Input: part model. Units: mm. Frame: model coordinates. Face numbers are marked on the shaded views. A direction names the side the tool comes from. Give positions to 0.01 mm unless a question says otherwise; leave off trailing zeros. Use a Markdown table: item, result. Add a question column.
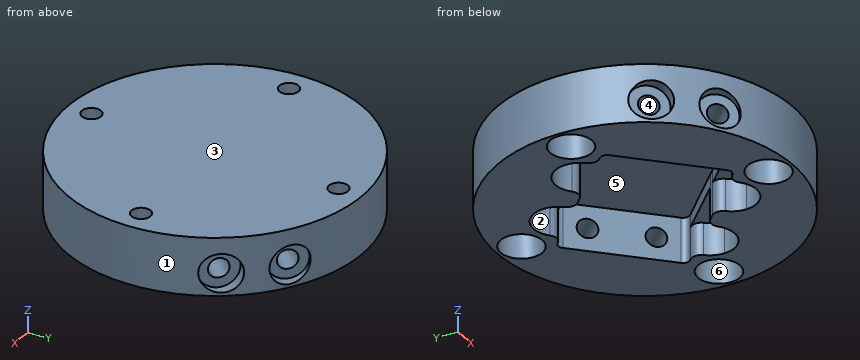
from build123d import *

# Parameters (mm, degrees)
SKETCH_1_R               = 23
SKETCH_1_R_2             = 1.5
EXTRUDE_1_DEPTH          = 7
FILLET_1_R               = 1.5
FILLET_2_R               = 1.5
EXTRUDE_2_DEPTH          = 2
FILLET_3_R               = 1
SKETCH_4_R               = 3.25
SKETCH_4_R_2             = 1.5
CUT_EXTRUDE_1_DEPTH      = 4
SKETCH_5_R               = 23
SKETCH_5_R_2             = 1.5
EXTRUDE_3_DEPTH          = 2
CUT_EXTRUDE_2_DEPTH      = 47.064665113
CUT_EXTRUDE_2_DEPTH_BACK = 47.064665113
SKETCH_6_R               = 1.5
SKETCH_7_R               = 3
SKETCH_7_R_2             = 1.5
CUT_EXTRUDE_3_DEPTH      = 2


with BuildPart() as part:
    # 草图1 → 凸台-拉伸1 (new body)
    with BuildSketch(Plane.XY):
        Circle(SKETCH_1_R)
        with Locations((-19.25, 0)):
            Circle(SKETCH_1_R_2, mode=Mode.SUBTRACT)
        with Locations((0, -19.25)):
            Circle(SKETCH_1_R_2, mode=Mode.SUBTRACT)
        with BuildLine():
            Line((0.386679311, 13.326733407), (2.474873734, 15.41492783))
            Line((2.474873734, 15.41492783), (15.41492783, 2.474873734))
            Line((15.41492783, 2.474873734), (13.326733407, 0.386679311))
            ThreePointArc((13.326733407, 0.386679311), (14.906146236, -1.051434667), (15.491109915, -3.105828541))
            ThreePointArc((15.491109915, -3.105828541), (12.482518738, -6.902589044), (8.098602063, -4.841452032))
            Line((8.098602063, -4.841452032), (4.841452032, -8.098602063))
            ThreePointArc((4.841452032, -8.098602063), (6.420864862, -9.536716041), (7.005828541, -11.591109915))
            ThreePointArc((7.005828541, -11.591109915), (3.997237363, -15.387870418), (-0.386679311, -13.326733407))
            Line((-0.386679311, -13.326733407), (-2.474873734, -15.41492783))
            Line((-2.474873734, -15.41492783), (-15.41492783, -2.474873734))
            Line((-15.41492783, -2.474873734), (-13.326733407, -0.386679311))
            ThreePointArc((-13.326733407, -0.386679311), (-14.348826362, 5.863544988), (-8.098602063, 4.841452032))
            Line((-8.098602063, 4.841452032), (-4.841452032, 8.098602063))
            ThreePointArc((-4.841452032, 8.098602063), (-5.863544988, 14.348826362), (0.386679311, 13.326733407))
        make_face(mode=Mode.SUBTRACT)
        with Locations((19.25, 0)):
            Circle(SKETCH_1_R_2, mode=Mode.SUBTRACT)
        with Locations((0, 19.25)):
            Circle(SKETCH_1_R_2, mode=Mode.SUBTRACT)
    extrude(amount=EXTRUDE_1_DEPTH)

    # 圆角1
    fillet_1_edges = [part.edges().sort_by_distance(p)[0] for p in [
        (0.386679311, 13.326733407, 3.5),
    ]]
    fillet(fillet_1_edges, radius=FILLET_1_R)

    # 圆角2
    fillet_2_edges = [part.edges().sort_by_distance(p)[0] for p in [
        (-4.841452032, 8.098602063, 3.5),
        (-8.098602063, 4.841452032, 3.5),
        (-13.326733407, -0.386679311, 3.5),
        (-0.386679311, -13.326733407, 3.5),
        (4.841452032, -8.098602063, 3.5),
        (8.098602063, -4.841452032, 3.5),
        (13.326733407, 0.386679311, 3.5),
    ]]
    fillet(fillet_2_edges, radius=FILLET_2_R)

    # 草图3 → 凸台-拉伸2 (add)
    with BuildSketch(Plane.XY.offset(7)):
        with BuildLine():
            Line((-14.526694033, -1.586639938), (-6.898641437, 6.041412659))
            ThreePointArc((-6.898641437, 6.041412659), (-7.923500416, 5.602500133), (-8.968137249, 5.992004973))
            ThreePointArc((-8.968137249, 5.992004973), (-14.348826362, 5.863544988), (-14.477286347, 0.482855875))
            ThreePointArc((-14.477286347, 0.482855875), (-14.087781508, -0.561780958), (-14.526694033, -1.586639938))
        make_face()
        with BuildLine():
            Line((-6.041412659, 6.898641437), (1.586639938, 14.526694033))
            ThreePointArc((1.586639938, 14.526694033), (0.561780958, 14.087781508), (-0.482855875, 14.477286347))
            ThreePointArc((-0.482855875, 14.477286347), (-5.863544988, 14.348826362), (-5.992004973, 8.968137249))
            ThreePointArc((-5.992004973, 8.968137249), (-5.602500133, 7.923500416), (-6.041412659, 6.898641437))
        make_face()
        with BuildLine():
            ThreePointArc((14.477286347, -0.482855875), (14.087781508, 0.561780958), (14.526694033, 1.586639938))
            Line((14.526694033, 1.586639938), (6.898641437, -6.041412659))
            ThreePointArc((6.898641437, -6.041412659), (7.923500416, -5.602500133), (8.968137249, -5.992004973))
            ThreePointArc((8.968137249, -5.992004973), (14.348826362, -5.863544988), (14.477286347, -0.482855875))
        make_face()
        with BuildLine():
            ThreePointArc((5.992004973, -8.968137249), (5.602500133, -7.923500416), (6.041412659, -6.898641437))
            Line((6.041412659, -6.898641437), (-1.586639938, -14.526694033))
            ThreePointArc((-1.586639938, -14.526694033), (-0.561780958, -14.087781508), (0.482855875, -14.477286347))
            ThreePointArc((0.482855875, -14.477286347), (5.863544988, -14.348826362), (5.992004973, -8.968137249))
        make_face()
    extrude(amount=-EXTRUDE_2_DEPTH)

    # 圆角3
    fillet_3_edges = [part.edges().sort_by_distance(p)[0] for p in [
        (-15.41492783, -2.474873734, 3.5),
        (-2.474873734, -15.41492783, 3.5),
        (15.41492783, 2.474873734, 3.5),
        (2.474873734, 15.41492783, 3.5),
    ]]
    fillet(fillet_3_edges, radius=FILLET_3_R)

    # 草图4 → 切除-拉伸1 (cut)
    # profile 1 of 4: a face of its own
    with BuildSketch(Plane(origin=(0, 0, 0), x_dir=(-1, 0, 0), z_dir=(0, 0, -1))):
        with Locations((-19.25, 0)):
            Circle(SKETCH_4_R)
        with Locations((-19.25, 0)):
            Circle(SKETCH_4_R_2, mode=Mode.SUBTRACT)
    # profile 2 of 4: a face of its own
    with BuildSketch(Plane(origin=(0, 0, 0), x_dir=(-1, 0, 0), z_dir=(0, 0, -1))):
        with Locations((0, 19.25)):
            Circle(SKETCH_4_R)
        with Locations((0, 19.25)):
            Circle(SKETCH_4_R_2, mode=Mode.SUBTRACT)
    # profile 3 of 4: a face of its own
    with BuildSketch(Plane(origin=(0, 0, 0), x_dir=(-1, 0, 0), z_dir=(0, 0, -1))):
        with Locations((19.25, 0)):
            Circle(SKETCH_4_R)
        with Locations((19.25, 0)):
            Circle(SKETCH_4_R_2, mode=Mode.SUBTRACT)
    # profile 4 of 4: a face of its own
    with BuildSketch(Plane(origin=(0, 0, 0), x_dir=(-1, 0, 0), z_dir=(0, 0, -1))):
        with Locations((0, -19.25)):
            Circle(SKETCH_4_R)
        with Locations((0, -19.25)):
            Circle(SKETCH_4_R_2, mode=Mode.SUBTRACT)
    extrude(amount=-CUT_EXTRUDE_1_DEPTH, mode=Mode.SUBTRACT)

    # 草图5 → 凸台-拉伸3 (add)
    with BuildSketch(Plane.XY.offset(7)):
        Circle(SKETCH_5_R)
        with Locations(Location((-19.25, 0, 0), (0, 0, 180))):
            Circle(SKETCH_5_R_2, mode=Mode.SUBTRACT)
        with Locations(Location((0, -19.25, 0), (0, 0, 180))):
            Circle(SKETCH_5_R_2, mode=Mode.SUBTRACT)
        with Locations(Location((19.25, 0, 0), (0, 0, 180))):
            Circle(SKETCH_5_R_2, mode=Mode.SUBTRACT)
        with Locations(Location((0, 19.25, 0), (0, 0, 180))):
            Circle(SKETCH_5_R_2, mode=Mode.SUBTRACT)
    extrude(amount=EXTRUDE_3_DEPTH)

    # 草图6 → 切除-拉伸2 (cut, two sides: drawn at the far end of the back side and taken through both)
    with BuildSketch(Plane(origin=(8.944900782, 8.944900782, 0), x_dir=(0, 0, 1), z_dir=(-0.7071067811865475, -0.7071067811865477, 0)).offset(-CUT_EXTRUDE_2_DEPTH_BACK)):
        with Locations(Location((3.5, 4.75, 0), (0, 0, 270))):
            Circle(SKETCH_6_R)
        with Locations(Location((3.5, -4.75, 0), (0, 0, 270))):
            Circle(SKETCH_6_R)
    extrude(amount=CUT_EXTRUDE_2_DEPTH + CUT_EXTRUDE_2_DEPTH_BACK, mode=Mode.SUBTRACT)

    # 草图7 → 切除-拉伸3 (cut)
    # profile 1 of 2: a face of its own
    with BuildSketch(Plane(origin=(-16.263455967, -16.263455967, 0), x_dir=(-0.7071067811865477, 0.7071067811865475, 0), z_dir=(-0.7071067811865475, -0.7071067811865477, 0))):
        with Locations(Location((-4.75, -3.5, 0), (0, 0, 180))):
            Circle(SKETCH_7_R)
        with Locations(Location((-4.75, -3.5, 0), (0, 0, 180))):
            Circle(SKETCH_7_R_2, mode=Mode.SUBTRACT)
    # profile 2 of 2: a face of its own
    with BuildSketch(Plane(origin=(-16.263455967, -16.263455967, 0), x_dir=(-0.7071067811865477, 0.7071067811865475, 0), z_dir=(-0.7071067811865475, -0.7071067811865477, 0))):
        with Locations(Location((4.75, -3.5, 0), (0, 0, 180))):
            Circle(SKETCH_7_R)
        with Locations(Location((4.75, -3.5, 0), (0, 0, 180))):
            Circle(SKETCH_7_R_2, mode=Mode.SUBTRACT)
    cut_extrude_3 = extrude(amount=-CUT_EXTRUDE_3_DEPTH, mode=Mode.SUBTRACT)

    # 镜向1: 切除-拉伸3 across plane
    add(cut_extrude_3.mirror(Plane(origin=(0, 0, 0), x_dir=(0, 0, 1), z_dir=(0.7071067811865476, 0.7071067811865476, 0))), mode=Mode.SUBTRACT)


solid = part.part
Q1. First-contact query: pin 1 (3.5 mm diameter, centred on x = -19.25, y = 0, fed in from -Z); pin 2 (3 mm diameter, centred on x = -18, z = 6, fed in from -Y); pin 3 (2.5 mm diameter, centred on x = 12.5, y = -1, fed in from -Z). Flat tips, straight axial feed; report the tip coordinate or a pass-through.
Q2. Access query for the marked faces 1 and 2. Directions: +Z, -Z, +X, -X, +Y, -Y. A direction counts if a zero-diameter tool reaches every point of the face in a straight line with its end or side. Return the directions, or none.
Q3. Draft query along Z for the marked faces 3, 4, 5 and 6. Return one class per face: +Z half, -Z half, draft (parallel to the pull), parting line (faces both ways), or undercut.
Q4. Ray query, line 1 (Y direction, x = 0, z = 7.65); line 2 (Y direction, x = 0, z = 2.8); line 3 (X direction, y = -6.5, z = 2.25). Return the intervals inside material, ascending.
Solution:
| question | item | result |
|---|---|---|
| 1 | pin 1 | stops at z = 4 |
| 1 | pin 2 | stops at y = -16.02 |
| 1 | pin 3 | stops at z = 5 |
| 2 | face 1 | +Z, -Z |
| 2 | face 2 | -Z |
| 3 | face 3 | +Z half |
| 3 | face 4 | undercut |
| 3 | face 5 | -Z half |
| 3 | face 6 | draft |
| 4 | line 1 | y = -23 to -20.75, -17.75 to 17.75, 20.75 to 23 |
| 4 | line 2 | y = -23 to -22.5, -16 to -14.18, 14.18 to 16, 22.5 to 23 |
| 4 | line 3 | x = -22.06 to -14.39, -12.04 to -11.39, 6.44 to 9.67, 13.51 to 22.06 |
